```python
from build123d import *

# Parameters (mm, degrees)
SKETCH_1_W      = 90
SKETCH_1_H      = 20
SKETCH_1_R      = 4.5
EXTRUDE_1_DEPTH = 16.25


with BuildPart() as part:
    # 草图1 → 凸台-拉伸1 (new body)
    with BuildSketch(Plane.XY):
        Rectangle(SKETCH_1_W, SKETCH_1_H)
        with Locations((-30, 0)):
            Circle(SKETCH_1_R, mode=Mode.SUBTRACT)
        Circle(SKETCH_1_R, mode=Mode.SUBTRACT)
        with Locations((30, 0)):
            Circle(SKETCH_1_R, mode=Mode.SUBTRACT)
    extrude(amount=EXTRUDE_1_DEPTH)


solid = part.part
```
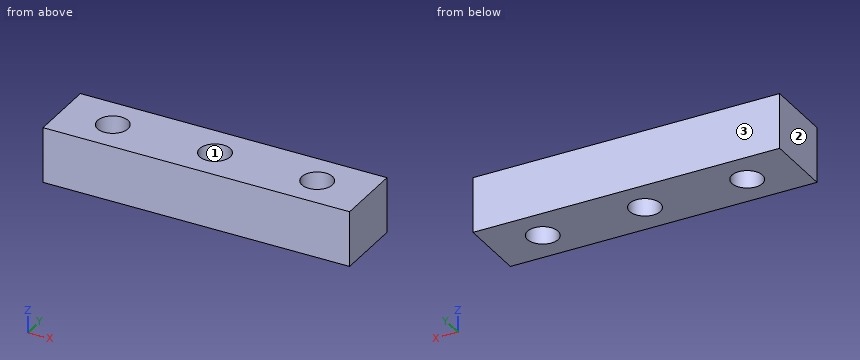
Geometry check sheet. Reference: the model listing, model coordinates, mm. Face numbers are marked on the shaded views. Coordinates: 2 decimals unless noted, no trailing zeros. Loops run counter-clockwise (first coordinate to the right, second up) from the corner with the lowest first, then second, coordinate; pieces in that order, holes last.
Item 1: Sectioned sample at C-C, the plane z = 1.25. Record the boundary of the cut face in (x, y), then the cut area to 3 significant figures.
Item 2: Release check for a two-part mould opening along X. For the marked faces 1, 2 and 3 record: released by +X, released by -X, zero draft, split by the parting line, or undercut.
Item 3: Sectioned sample at B-B, the plane x = -30. Record the boundary of the cut face in (y, z).
Item 4: Go/stop test with a flat-tipped pin: pin 1 Ø5.5 at (x, y) = (-30, 0) entering from -Z. Record where the tip stops, or that it passes through.
Item 5: Thickness scan on line 1 (Y direction, x = 0, z = 8); line 2 (X direction, y = -3.75, z = 5); line 3 (X direction, y = 4, z = 1.25). Record the ranges inside material, lowest first.
Item 6: Sectioned sample at A-A, the plane y = 0. Record the boundary of the cut face in (x, z).
Check result:
1. outline: (-45, -10) - (45, -10) - (45, 10) - (-45, 10) - close; hole circle Ø9 at (-30, 0); hole circle Ø9 at (0, 0); hole circle Ø9 at (30, 0)
1. area: 1,610 mm2
2. face 1: undercut
2. face 2: released by -X
2. face 3: zero draft
3. outline: (-10, 0) - (-4.5, 0) - (-4.5, 16.25) - (-10, 16.25) - close; (4.5, 0) - (10, 0) - (10, 16.25) - (4.5, 16.25) - close
4. pin 1: passes through
5. line 1: y = -10 to -4.5, 4.5 to 10
5. line 2: x = -45 to -32.49, -27.51 to -2.49, 2.49 to 27.51, 32.49 to 45
5. line 3: x = -45 to -32.06, -27.94 to -2.06, 2.06 to 27.94, 32.06 to 45
6. outline: (-45, 0) - (-34.5, 0) - (-34.5, 16.25) - (-45, 16.25) - close; (-25.5, 0) - (-4.5, 0) - (-4.5, 16.25) - (-25.5, 16.25) - close; (4.5, 0) - (25.5, 0) - (25.5, 16.25) - (4.5, 16.25) - close; (34.5, 0) - (45, 0) - (45, 16.25) - (34.5, 16.25) - close
